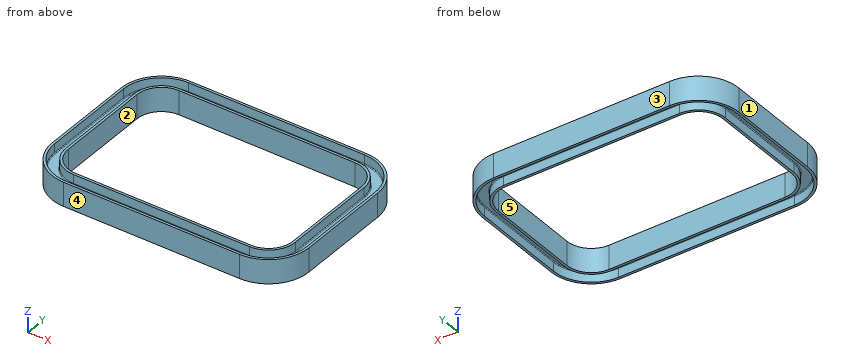
```python
from build123d import *


with BuildPart() as f2:
    # F2: sweep along a path in F0
    with BuildLine(Plane.XY) as f2_path:
        Line((55, 50), (-55, 50))
        ThreePointArc((-55, 50), (-69.142136, 44.142136), (-75, 30))
        Line((-75, 30), (-75, -30))
        ThreePointArc((-75, -30), (-69.142136, -44.142136), (-55, -50))
        Line((-55, -50), (55, -50))
        ThreePointArc((55, -50), (69.142136, -44.142136), (75, -30))
        Line((75, -30), (75, 30))
        ThreePointArc((75, 30), (69.142136, 44.142136), (55, 50))
    # F1 (on Right) → F2 (sweep)
    with BuildSketch(Plane.YZ):
        with BuildLine():
            Line((55.19626, 0), (55.19626, 7.5))
            Line((55.19626, 7.5), (53.69626, 7.5))
            Line((53.69626, 7.5), (53.69626, 2))
            ThreePointArc((53.69626, 2), (53.549814, 1.646447), (53.19626, 1.5))
            Line((53.19626, 1.5), (47.19626, 1.5))
            ThreePointArc((47.19626, 1.5), (46.842707, 1.646447), (46.69626, 2))
            Line((46.69626, 2), (46.69626, 7.5))
            Line((46.69626, 7.5), (45.19626, 7.5))
            Line((45.19626, 7.5), (45.19626, -7.5))
            Line((45.19626, -7.5), (46.69626, -7.5))
            Line((46.69626, -7.5), (46.69626, -2))
            ThreePointArc((46.69626, -2), (46.842707, -1.646447), (47.19626, -1.5))
            Line((47.19626, -1.5), (53.19626, -1.5))
            ThreePointArc((53.19626, -1.5), (53.549814, -1.646447), (53.69626, -2))
            Line((53.69626, -2), (53.69626, -7.5))
            Line((53.69626, -7.5), (55.19626, -7.5))
            Line((55.19626, -7.5), (55.19626, 0))
        make_face()
    sweep(path=f2_path.line)


solid = f2.part
```
Source: CAD feature listing. Evaluate the final solid. Frame: model axes, mm. Face numbers are marked on the shaded views. A direction names the side the tool comes from. Give positions to 0.01 mm unless a question says otherwise; leave off trailing zeros. Use a Markdown table: item, result. Add a question column.
(1) Pull-direction query (Y, two-part tool) for the marked faces 3, 4 and 5; classes: +Y half, -Y half, draft (parallel to the pull), parting line (faces both ways), or undercut.
(2) Section query A-A (z = -4.75). Count the separate pieces of the cut face and the enclosed holes in it, then the cut area to 3 significant figures.
(3) Ray query, line 1 (Y direction, x = -28.5, z = -3); line 2 (X direction, y = -7, z = 5.25); line 3 (Y direction, x = -57, z = 7). Return the intervals inside material, ascending.
(4) Access query for the marked faces 1 and 2. Directions: +Z, -Z, +X, -X, +Y, -Y. A direction counts if a zero-diameter tool reaches every point of the face in a straight line with its end or side. Return the directions, or none.
Checked values:
| question | item | result |
|---|---|---|
| 1 | face 3 | +Y half |
| 1 | face 4 | -Y half |
| 1 | face 5 | undercut |
| 2 | separate pieces | 2 |
| 2 | enclosed holes | 2 |
| 2 | area | 1,400 mm^2 |
| 3 | line 1 | -55.2 to -53.7, -46.7 to -45.2, 45.2 to 46.7, 53.7 to 55.2 |
| 3 | line 2 | -80.2 to -78.7, -71.7 to -70.2, 70.2 to 71.7, 78.7 to 80.2 |
| 3 | line 3 | -55.12 to -53.61, -46.58 to -45.06, 45.06 to 46.58, 53.61 to 55.12 |
| 4 | face 1 | +Z, -Z, -X, +Y, -Y |
| 4 | face 2 | +Z, -Z |
